```python
from build123d import *

# Parameters (mm, degrees)
F1_DEPTH = 5.08
F2_DEPTH = 25.4
F3_DEPTH = 17.78


with BuildPart() as f1:
    # F0 (on Front) → F1 (new body)
    with BuildSketch(Plane.XZ):
        with BuildLine():
            ThreePointArc((-27.94, 0), (-29.4278975516, 3.5921024484), (-33.02, 5.08))
            ThreePointArc((-33.02, 5.08), (-36.6121024484, 3.5921024484), (-38.1, 0))
            ThreePointArc((-38.1, 0), (-36.6121024484, -3.5921024484), (-33.02, -5.08))
            ThreePointArc((-33.02, -5.08), (-29.4278975516, -3.5921024484), (-27.94, 0))
        make_face()
        with BuildLine():
            Line((33.019999962, 5.08), (-33.02, 5.08))
            ThreePointArc((-33.02, 5.08), (-29.4278975516, 3.5921024484), (-27.94, 0))
            ThreePointArc((-27.94, 0), (-29.4278975516, -3.5921024484), (-33.02, -5.08))
            Line((-33.02, -5.08), (33.02, -5.08))
            ThreePointArc((33.02, -5.08), (27.94, -1.9e-08), (33.019999962, 5.08))
        make_face()
        with BuildLine():
            ThreePointArc((38.1, 0), (36.612102435, 3.5921024619), (33.019999962, 5.08))
            ThreePointArc((33.019999962, 5.08), (27.94, -1.9e-08), (33.02, -5.08))
            ThreePointArc((33.02, -5.08), (36.6121024484, -3.5921024484), (38.1, 0))
        make_face()
    extrude(amount=-F1_DEPTH)

    # F0 (on Front) → F2 (join)
    with BuildSketch(Plane.XZ):
        with BuildLine():
            ThreePointArc((-27.94, 0), (-29.4278975516, 3.5921024484), (-33.02, 5.08))
            ThreePointArc((-33.02, 5.08), (-36.6121024484, 3.5921024484), (-38.1, 0))
            ThreePointArc((-38.1, 0), (-36.6121024484, -3.5921024484), (-33.02, -5.08))
            ThreePointArc((-33.02, -5.08), (-29.4278975516, -3.5921024484), (-27.94, 0))
        make_face()
    extrude(amount=F2_DEPTH)

    # F0 (on Front) → F3 (join)
    with BuildSketch(Plane.XZ):
        with BuildLine():
            ThreePointArc((38.1, 0), (36.612102435, 3.5921024619), (33.019999962, 5.08))
            ThreePointArc((33.019999962, 5.08), (27.94, -1.9e-08), (33.02, -5.08))
            ThreePointArc((33.02, -5.08), (36.6121024484, -3.5921024484), (38.1, 0))
        make_face()
    extrude(amount=-F3_DEPTH)


solid = f1.part
```
Can you work these out from the model? Positions are in its coordinate system, mm. A direction names the side the tool comes from. Round coordinates to 2 decimals unless told otherwise and drop trailing zeros. Loops run counter-clockwise (first coordinate to the right, second up) from the corner with the lowest first, then second, coordinate; pieces in that order, holes last. Notation, with made-up numbers: M 67,84 L 120,84 A21 ccw 120,109 Z; hole C 12,18.5 d5. An arc over 180 degrees is marked long. Answer as a JSON object with one key per item and string values. Group by question number.
Q1. We'd pull the mould along X, two halves only. Please class faces 1 (the cylindrical face through (38, 11, 1)), 2 (the flat face through (-33, -25.4, 0)): +X half, -X half, draft (parallel to the pull), parting line (faces both ways), or undercut.
Q2. Will these pins go through, and if not, where does the flat tip stop? pin 1 (2 mm diameter, centred on x = 12.5, z = 1, fed in from +Y); pin 2 (5 mm diameter, centred on x = 14.5, y = 7, fed in from -Z); pin 3 (6 mm diameter, centred on x = 1, z = 3.5, fed in from -Y); pin 4 (6 mm diameter, centred on y = -4, z = 1, fed in from +X).
Q3. On a 3-axis mill with a long thin cutter (end or side, diameter ignored), from which of +Z, -Z, +X, -X, +Y, -Y can I reach the whole of each face in a straight line? I mean faces 3 (the flat face through (33, 17.78, 0)), 4 (the cylindrical face through (-38.095, -9.947, 0.223)). Say none if no direction works.
Q4. Imagine slicing it at D-D, the plane y = 1.5. Please give me the cut outline in (x, z).
Q5. Please list where these lines run through material, in increasing order: L1, parallel to Y at x = 30, z = 3.25; L2, parallel to Y at x = 3.5, z = 4.75; L3, parallel to X at y = 1.5, z = 2.25.
Q6. Imagine slicing it at A-A, the plane z = 0. Please give me the cut outline in (x, y).
Q7. Imagine slicing it at B-B, the plane x = 31. Please give me the cut outline in (y, z), then the cut area to 3 significant figures.
Q8. Imagine slicing it at C-C, the plane y = -9.5. Please give me the cut outline in (x, z).
Findings:
{
 "1": {"face 1": "parting line", "face 2": "draft"},
 "2": {"pin 1": "stops at y = 5.08", "pin 2": "stops at z = -5.08", "pin 3": "stops at y = 0", "pin 4": "stops at x = -27.94"},
 "3": {"face 3": "+Z, -Z, +X, -X, +Y", "face 4": "-Y"},
 "4": {"outline": "M -33.02,-5.08 L 33.02,-5.08 A5.08 ccw 33.02,5.08 L -33.02,5.08 A5.08 ccw Z"},
 "5": {"L1": "y = 0 to 17.78", "L2": "y = 0 to 5.08", "L3": "x = -37.57 to 37.57"},
 "6": {"outline": "M -38.1,-25.4 L -27.94,-25.4 L -27.94,0 L 38.1,0 L 38.1,17.78 L 27.94,17.78 L 27.94,5.08 L -38.1,5.08 Z"},
 "7": {"outline": "M 0,-5.08 L 5.08,-5.08 L 5.08,-4.66 L 17.78,-4.66 L 17.78,4.66 L 5.08,4.66 L 5.08,5.08 L 0,5.08 Z", "area": "170 mm2"},
 "8": {"outline": "C -33.02,0 d10.16"}
}
